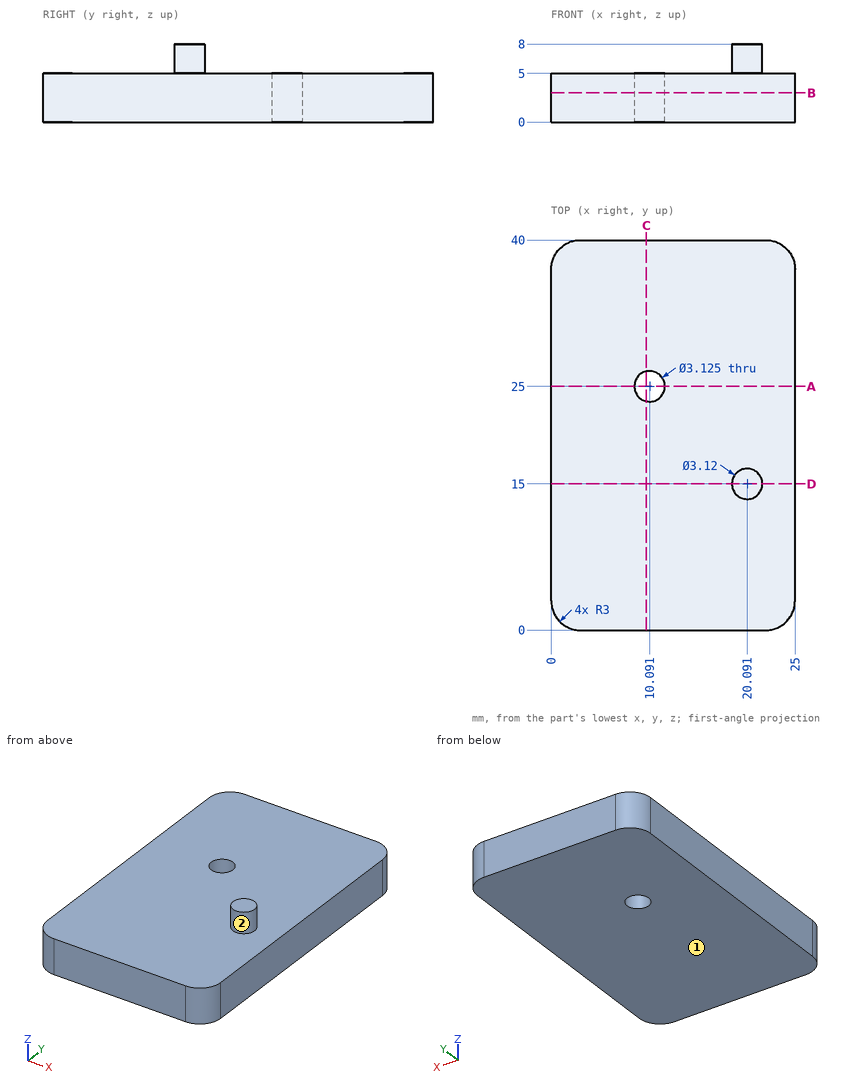
Verification items for this drawing (mm, ordinates from the low corner). A direction names the side the tool comes from. Coordinates: 2 decimals unless noted, no trailing zeros. Loops run counter-clockwise (first coordinate to the right, second up) from the corner with the lowest first, then second, coordinate; pieces in that order, holes last. Notation, with made-up numbers: (21, 72) -> (45, 72) arc R4 cw to (45, 77) -> close; hole circle Ø5 at (73.25, -33.5). An arc over 180 degrees is marked (long way). Put each result on its own line as item: value.
1. Section check B-B, the plane z = 3. Record the boundary of the cut face in (x, y) (1 decimal), then the cut area to 3 significant figures.
Result set:
outline: (0, 3) arc R3 ccw to (3, 0) -> (22, 0) arc R3 ccw to (25, 3) -> (25, 37) arc R3 ccw to (22, 40) -> (3, 40) arc R3 ccw to (0, 37) -> close; hole circle Ø3.1 at (10.1, 25)
area: 985 mm^2
2. Section check C-C, the plane x = 9.75. Record the boundary of the cut face in (y, z) (3 decimals), then the cut area to 3 significant figures.
Result set:
outline: (0, 0) -> (23.475, 0) -> (23.475, 5) -> (0, 5) -> close; (26.525, 0) -> (40, 0) -> (40, 5) -> (26.525, 5) -> close
area: 185 mm^2
3. Gauge pin test, flat end, axial feed: P1, Ø12, axis at x = 22.5, y = 26, coming from the +Z side. Record the tip position at first contact, or that the pin passes through.
Result set:
P1: stops at z = 5
4. Section check A-A, the plane y = 25. Record the boundary of the cut face in (x, z), then the cut area to 3 significant figures.
Result set:
outline: (0, 0) -> (8.53, 0) -> (8.53, 5) -> (0, 5) -> close; (11.65, 0) -> (25, 0) -> (25, 5) -> (11.65, 5) -> close
area: 109 mm^2
5. Tool access check on the marked faces 1 and 2. Record the directions out of +Z, -Z, +X, -X, +Y, -Y that give a thin tool (end or side, any length) a straight path to the whole face; none if there is none.
Result set:
face 1: -Z, +X, -X, +Y, -Y
face 2: +Z
6. Thickness scan on line 1 (Z direction, x = 4.5, y = 35.5). Record the ranges inside material, lowest first.
Result set:
line 1: z = 0 to 5
7. Section check D-D, the plane y = 15. Record the boundary of the cut face in (x, z), then the cut area to 3 significant figures.
Result set:
outline: (0, 0) -> (25, 0) -> (25, 5) -> (21.65, 5) -> (21.65, 8) -> (18.53, 8) -> (18.53, 5) -> (0, 5) -> close
area: 134 mm^2
